```python
from build123d import *

# Parameters (mm, degrees)
CYLINDER_R       = 24.765
CYLINDER_DEPTH   = 19.05
HOLE_D           = 4.1
HOLE_DEPTH       = 14.986
HOLE_CSINK_D     = 5.207
HOLE_CSINK_ANGLE = 90
HOLE_TIPS_R      = 2.05
SKETCH001_R      = 14.2875
POCKET_DEPTH     = 12.7
SKETCH002_R      = 16.764
SKETCH002_R_2    = 14.986
POCKET001_DEPTH  = 1.6002
CHAMFER_SIZE     = 0.254


with BuildPart() as part:
    # Cylinder → Cylinder (join)
    with BuildSketch(Plane.XY):
        Circle(CYLINDER_R)
    extrude(amount=CYLINDER_DEPTH)

    # Hole
    with Locations(Plane.XY.offset(19.05)):
        with Locations((0, 20.6502), (17.883598, 10.3251), (17.883598, -10.3251), (0, -20.6502), (-17.883598, -10.3251), (-17.883598, 10.3251)):
            CounterSinkHole(HOLE_D / 2, HOLE_CSINK_D / 2, depth=HOLE_DEPTH, counter_sink_angle=HOLE_CSINK_ANGLE)

    # Hole tips → Hole tip 1 section 0
    with BuildSketch(Plane.XY.offset(4.064), mode=Mode.PRIVATE) as hole_tip_1_s0:
        with Locations((0, 20.6502)):
            Circle(HOLE_TIPS_R)
    loft([hole_tip_1_s0.sketch, Vertex(0, 20.6502, 2.832236)], mode=Mode.SUBTRACT)

    # Hole tips → Hole tip 2 section 0
    with BuildSketch(Plane.XY.offset(4.064), mode=Mode.PRIVATE) as hole_tip_2_s0:
        with Locations((17.883598, 10.3251)):
            Circle(HOLE_TIPS_R)
    loft([hole_tip_2_s0.sketch, Vertex(17.883598, 10.3251, 2.832236)], mode=Mode.SUBTRACT)

    # Hole tips → Hole tip 3 section 0
    with BuildSketch(Plane.XY.offset(4.064), mode=Mode.PRIVATE) as hole_tip_3_s0:
        with Locations((17.883598, -10.3251)):
            Circle(HOLE_TIPS_R)
    loft([hole_tip_3_s0.sketch, Vertex(17.883598, -10.3251, 2.832236)], mode=Mode.SUBTRACT)

    # Hole tips → Hole tip 4 section 0
    with BuildSketch(Plane.XY.offset(4.064), mode=Mode.PRIVATE) as hole_tip_4_s0:
        with Locations((0, -20.6502)):
            Circle(HOLE_TIPS_R)
    loft([hole_tip_4_s0.sketch, Vertex(0, -20.6502, 2.832236)], mode=Mode.SUBTRACT)

    # Hole tips → Hole tip 5 section 0
    with BuildSketch(Plane.XY.offset(4.064), mode=Mode.PRIVATE) as hole_tip_5_s0:
        with Locations((-17.883598, -10.3251)):
            Circle(HOLE_TIPS_R)
    loft([hole_tip_5_s0.sketch, Vertex(-17.883598, -10.3251, 2.832236)], mode=Mode.SUBTRACT)

    # Hole tips → Hole tip 6 section 0
    with BuildSketch(Plane.XY.offset(4.064), mode=Mode.PRIVATE) as hole_tip_6_s0:
        with Locations((-17.883598, 10.3251)):
            Circle(HOLE_TIPS_R)
    loft([hole_tip_6_s0.sketch, Vertex(-17.883598, 10.3251, 2.832236)], mode=Mode.SUBTRACT)

    # Sketch001 (on Face2 of Hole) → Pocket (cut)
    with BuildSketch(Plane.XY.offset(19.05)):
        Circle(SKETCH001_R)
    extrude(amount=-POCKET_DEPTH, mode=Mode.SUBTRACT)

    # Sketch002 (on Face2 of Pocket) → Pocket001 (cut)
    with BuildSketch(Plane.XY.offset(19.05)):
        Circle(SKETCH002_R)
        Circle(SKETCH002_R_2, mode=Mode.SUBTRACT)
    extrude(amount=-POCKET001_DEPTH, mode=Mode.SUBTRACT)

    # Chamfer
    chamfer_edges = [part.edges().sort_by_distance(p)[0] for p in [
        (-14.2875, 0, 19.05),
        (-24.765, 0, 19.05),
        (-24.765, 0, 0),
    ]]
    chamfer(chamfer_edges, length=CHAMFER_SIZE)


solid = part.part
```
Read the model definition and answer for the solid it produces. Units are mm, in the model's axes. A direction names the side the tool comes from. Give positions to 0.01 mm unless a question says otherwise; leave off trailing zeros. Put each result on its own line as item: value. Start each with the question number.
1. Each of these flat-tipped pins is pushed along its axis until it touches: pin 1 Ø4 at (x, z) = (10, 10.5) entering from -Y; pin 2 Ø1 at (y, z) = (10.5, 5.5) entering from -X; pin 3 Ø2.5 at (x, y) = (17.88, -10.33) entering from +Z. Where does it stop, or does it pass through?
2. The part is cut by section A-A, the plane z = 8.5. Give the number of separate pieces and of enclosed holes in the cut face, and give its area (3 significant figures).
3. Which of the six approach directions +Z, -Z, +X, -X, +Y, -Y give full straight-line access (tool end or side, diameter ignored) to faces 1 (the flat face through (0, 0, 0)), 2 (the cylindrical face through (-14.274, 0.628, 12.66))?
4. For a pull along Y with two mould halves and no side action, classify faces 3 (the conical face through (17.62, 10.13, 3.03)), 4 (the flat face through (16, 6, 19.05)) as released by +Y, released by -Y, zero draft, split by the parting line, or undercut.
5. Consider line 1 along Y through (x, z) = (0, 18.15) (1 decimal); line 2 along Y through (x, z) = (17.5, 7.75); line 3 along Y through (x, z) = (-16, 15.5). Determine where each line is inside the solid, lowest interval first.
Final values:
1. pin 1: stops at y = -23.44
1. pin 2: stops at x = -22.66
1. pin 3: stops at z = 3.59
2. separate pieces: 1
2. enclosed holes: 7
2. area: 1,210 mm²
3. face 1: -Z, +X, -X, +Y, -Y
3. face 2: +Z
4. face 3: undercut
4. face 4: zero draft
5. line 1: y = -24.8 to -22.7, -18.6 to -16.8, -15 to -14.3, 14.3 to 15, 16.8 to 18.6, 22.7 to 24.8
5. line 2: y = -17.52 to -12.34, -8.31 to 8.31, 12.34 to 17.52
5. line 3: y = -18.9 to -11.13, -9.52 to 9.52, 11.13 to 18.9
